Here's how the part is built. I have some questions about the finished solid (model axes, mm). A direction names the side the tool comes from. Round coordinates to 2 decimals unless told otherwise and drop trailing zeros. Order: outer loops, then holes, each group sorted by start corner. A loop starts at its lowest first (then second) coordinate and runs counter-clockwise, first axis right, second up. Notation, with made-up numbers: (-39.75, 48) -> (-5.75, 48) arc R24 ccw to (-5.75, 67) -> close; hole circle Ø10 at (-34, 64.25). An arc over 180 degrees is marked (long way). Use a Markdown table: item, result. Add a question column.
from build123d import *

# Parameters (mm, degrees)
SKETCH1_W           = 100
SKETCH1_H           = 18
BOSS_EXTRUDE1_DEPTH = 18


with BuildPart() as part:
    # Sketch1 → Boss-Extrude1 (new body)
    with BuildSketch(Plane(origin=(0, 0, 0), x_dir=(1, 0, 0), z_dir=(0, 1, 0))):
        Polygon((-300, -7.111898923), (300, -7.111898923), (300, -13.111898923), (318, -13.111898923), (318, -113.111898923), (300, -113.111898923), (300, -601.111898923), (318, -601.111898923), (318, -701.111898923), (300, -701.111898923), (300, -707.111898923), (-300, -707.111898923), (-300, -701.111898923), (-318, -701.111898923), (-318, -601.111898923), (-300, -601.111898923), (-300, -113.111898923), (-318, -113.111898923), (-318, -13.111898923), (-300, -13.111898923), align=None)
        with Locations((-145, -692.111898923)):
            Rectangle(SKETCH1_W, SKETCH1_H, mode=Mode.SUBTRACT)
        with Locations((145, -692.111898923)):
            Rectangle(SKETCH1_W, SKETCH1_H, mode=Mode.SUBTRACT)
        with Locations((145, -492.111898923)):
            Rectangle(SKETCH1_W, SKETCH1_H, mode=Mode.SUBTRACT)
        with Locations((-145, -492.111898923)):
            Rectangle(SKETCH1_W, SKETCH1_H, mode=Mode.SUBTRACT)
        with Locations((145, -292.111898923)):
            Rectangle(SKETCH1_W, SKETCH1_H, mode=Mode.SUBTRACT)
        with Locations((-145, -292.111898923)):
            Rectangle(SKETCH1_W, SKETCH1_H, mode=Mode.SUBTRACT)
        with Locations((145, -92.111898923)):
            Rectangle(SKETCH1_W, SKETCH1_H, mode=Mode.SUBTRACT)
        with Locations((-145, -92.111898923)):
            Rectangle(SKETCH1_W, SKETCH1_H, mode=Mode.SUBTRACT)
    extrude(amount=BOSS_EXTRUDE1_DEPTH)


solid = part.part
(1) I want a section at B-B on y = 4.75. State how many separate pieces and enclosed holes the cut face has, and give its area (3 significant figures).
(2) I want a section at A-A on x = -178. List the corners of the cut face in (y, z) for me.
(3) If we mould it in two halves opening along Z, with no side actions, what happens to faces 1 (the flat face through (4, 9, 707.112)), 2 (the flat face through (4, 0, 352)), 3 (the flat face through (-300, 9, 361))? For each: pulls with the +Z half, pulls with the -Z half, needs draft (parallel to the pull), parting line crosses it, or undercut.
(4) On a 3-axis mill with a long thin cutter (end or side, diameter ignored), from which of +Z, -Z, +X, -X, +Y, -Y can I reach the whole of each face in a straight line? I mean faces 4 (the flat face through (95, 9, 92)), 5 (the flat face through (-309, 9, 13.112)), 6 (the flat face through (-309, 9, 113.112)). Say none if no direction works.
(5) I'm going to push flat-ended pins straight in: P1, Ø9, axis at y = 9, z = 290, coming from the -X side; P2, Ø1.5, axis at y = 11, z = 398, coming from the +X side; P3, Ø5.5, axis at x = -312.5, y = 12, coming from the +Z side. Where does each tip first touch, or does it pass through?
(6) Please list where these lines run through material, in increasing order: probe 1 along Z at (x, y) = (-174, 5.25); probe 2 along X at (y, z) = (1.25, 95.5); probe 3 along X at (y, z) = (15.5, 156.5). Write a range as from..to.
(7) I want a section at C-C on z = 327. List the corners of the cut face in (x, y) for me.
Output:
| question | item | result |
|---|---|---|
| 1 | separate pieces | 1 |
| 1 | enclosed holes | 8 |
| 1 | area | 413,000 mm² |
| 2 | outline | (0, 7.11) -> (18, 7.11) -> (18, 83.11) -> (0, 83.11) -> close; (0, 101.11) -> (18, 101.11) -> (18, 283.11) -> (0, 283.11) -> close; (0, 301.11) -> (18, 301.11) -> (18, 483.11) -> (0, 483.11) -> close; (0, 501.11) -> (18, 501.11) -> (18, 683.11) -> (0, 683.11) -> close; (0, 701.11) -> (18, 701.11) -> (18, 707.11) -> (0, 707.11) -> close |
| 3 | face 1 | pulls with the +Z half |
| 3 | face 2 | needs draft |
| 3 | face 3 | undercut |
| 4 | face 4 | +Y, -Y |
| 4 | face 5 | -Z, -X, +Y, -Y |
| 4 | face 6 | -X, +Y, -Y |
| 5 | P1 | x = -300 |
| 5 | P2 | x = 300 |
| 5 | P3 | z = 701.11 |
| 6 | probe 1 | 7.11..83.11, 101.11..283.11, 301.11..483.11, 501.11..683.11, 701.11..707.11 |
| 6 | probe 2 | -318..-195, -95..95, 195..318 |
| 6 | probe 3 | -300..300 |
| 7 | outline | (-300, 0) -> (300, 0) -> (300, 18) -> (-300, 18) -> close |
